from build123d import *

# Parameters (mm, degrees)
SKETCH2_R           = 14
BOSS_EXTRUDE1_DEPTH = 70
SKETCH3_R           = 11
CUT_EXTRUDE1_DEPTH  = 71
SKETCH4_W           = 32.230614228
SKETCH4_H           = 15.278665706
CUT_EXTRUDE2_DEPTH  = 71
SKETCH5_W           = 3
SKETCH5_H           = 8.740769075
BOSS_EXTRUDE3_DEPTH = 70
SKETCH7_R           = 2.5
CUT_EXTRUDE3_DEPTH  = 15


with BuildPart() as part:
    # Sketch2 → Boss-Extrude1 (new body)
    with BuildSketch(Plane.XY):
        Circle(SKETCH2_R)
    extrude(amount=BOSS_EXTRUDE1_DEPTH)

    # Sketch3 → Cut-Extrude1 (cut, through all)
    with BuildSketch(Plane.XY.offset(70)):
        Circle(SKETCH3_R)
    extrude(amount=-CUT_EXTRUDE1_DEPTH, mode=Mode.SUBTRACT)

    # Sketch4 → Cut-Extrude2 (cut, through all)
    with BuildSketch(Plane.XY.offset(70)):
        with Locations((0.085938844, 7.639332853)):
            Rectangle(SKETCH4_W, SKETCH4_H)
    extrude(amount=-CUT_EXTRUDE2_DEPTH, mode=Mode.SUBTRACT)

    # Sketch5 → Boss-Extrude3 (add)
    with BuildSketch(Plane.XY.offset(70)):
        with Locations((-12.5, 4.370384538)):
            Rectangle(SKETCH5_W, SKETCH5_H)
    extrude(amount=-BOSS_EXTRUDE3_DEPTH)

    # Sketch7 → Cut-Extrude3 (cut, through all)
    with BuildSketch(Plane(origin=(0, 0, 0), x_dir=(1, 0, 0), z_dir=(0, 1, 0))):
        with Locations((0, -38)):
            Circle(SKETCH7_R)
    extrude(amount=-CUT_EXTRUDE3_DEPTH, mode=Mode.SUBTRACT)


solid = part.part
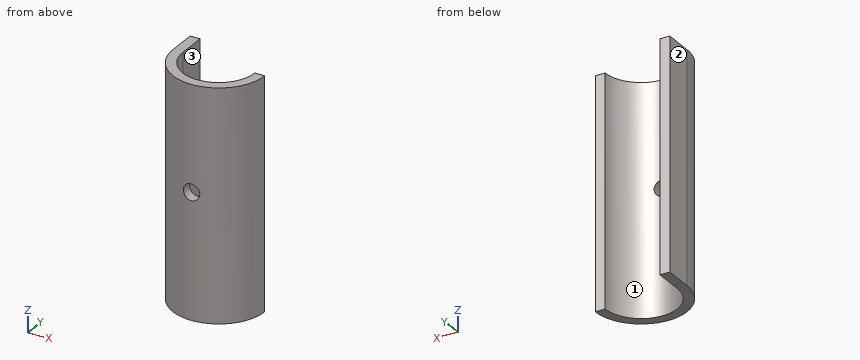
Geometry: final body of the model. Coordinates: model frame, mm. Face numbers are marked on the shaded views. Give positions to 0.01 mm unless a question says otherwise; leave off trailing zeros. Order: outer loops, then holes, each group sorted by start corner. A loop starts at its lowest first (then second) coordinate and runs counter-clockwise, first axis right, second up. Notation, with made-up numbers: (74.5, 31) -> (115.5, 31) arc R30 ccw to (115.5, 70) -> close; hole circle Ø1 at (68.5, 2.5). An arc over 180 degrees is marked (long way). Write each question's results on one line, items separated by ' | '.
1) Cut plane B-B (y = -8.5). Output: boundary loops of the cut face in (x, z).
Geometry says:
outline: (-11.12, 0) -> (-6.98, 0) -> (-6.98, 70) -> (-11.12, 70) -> close; (6.98, 0) -> (11.12, 0) -> (11.12, 70) -> (6.98, 70) -> close
2) Line query: line 1 along Z through (x, y) = (0, -11.4); line 2 along X through (y, z) = (-11.4, 38); line 3 along X through (y, z) = (-9, 41). Output: solid intervals per line, ascending.
Geometry says:
line 1: z = 0 to 35.5, 40.5 to 70 | line 2: x = -8.13 to -2.5, 2.5 to 8.13 | line 3: x = -10.72 to -6.32, 6.32 to 10.72
3) Cut plane D-D (z = 27). Output: boundary loops of the cut face in (x, y).
Geometry says:
outline: (-14, 0) arc R14 ccw to (14, 0) -> (11, 0) arc R11 cw to (-11, 0) -> (-11, 8.74) -> (-14, 8.74) -> close
4) Cut plane C-C (z = 38). Output: boundary loops of the cut face in (x, y).
Geometry says:
outline: (-14, 0) arc R14 ccw to (-2.5, -13.77) -> (-2.5, -10.71) arc R11 cw to (-11, 0) -> (-11, 8.74) -> (-14, 8.74) -> close; (2.5, -13.77) arc R14 ccw to (14, 0) -> (11, 0) arc R11 cw to (2.5, -10.71) -> close
5) First-contact query: pin 1 Ø12 at (x, y) = (-8, -1) entering from -Z; pin 2 Ø2.5 at (y, z) = (5, 49.5) entering from +X; pin 3 Ø5 at (x, z) = (-10, 14) entering from -Y; pin 4 Ø1.5 at (x, z) = (12.5, 28.5) entering from +Y. Flat tips, straight axial feed; report the tip coordinate or a pass-through.
Geometry says:
pin 1: stops at z = 0 | pin 2: stops at x = -11 | pin 3: stops at y = -11.82 | pin 4: stops at y = 0
6) Draft query along X for the marked faces 1, 2 and 3. Return one class per face: released by +X, released by -X, zero draft, split by the parting line, or undercut.
Geometry says:
face 1: undercut | face 2: released by -X | face 3: released by +X
7) Cut plane A-A (x = 0). Output: boundary loops of the cut face in (y, z), and give its area (3 significant figures).
Geometry says:
outline: (-14, 0) -> (-11, 0) -> (-11, 35.5) -> (-14, 35.5) -> close; (-14, 40.5) -> (-11, 40.5) -> (-11, 70) -> (-14, 70) -> close | area: 195 mm²
